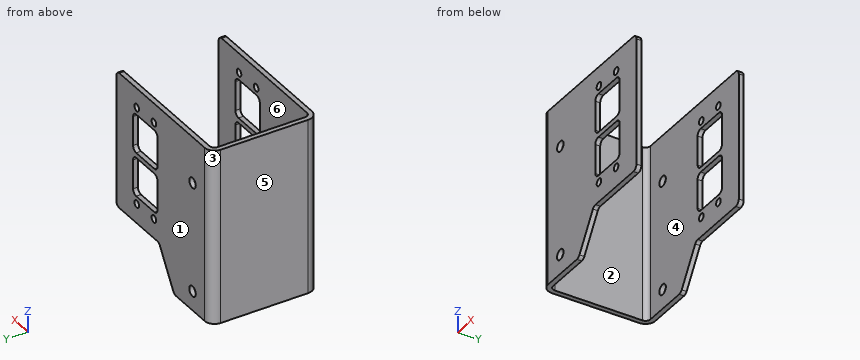
```python
from build123d import *

# Parameters (mm, degrees)
SKETCH1_W                      = 114.3
SKETCH1_H                      = 69.85
BASE_FLANGE1_DEPTH             = 3.175
EDGE_FLANGE1_STRIP_W           = 19.05
EDGE_FLANGE1_STRIP_H           = 3.175
EDGE_FLANGE1_STRIP_CUT_DEPTH   = 114.3
EDGE_FLANGE1_STRIP_2_W         = 19.05
EDGE_FLANGE1_STRIP_2_H         = 3.175
EDGE_FLANGE1_STRIP_CUT_2_DEPTH = 114.3
EDGE_FLANGE1_DEPTH             = 114.3
EDGE_FLANGE1_BEND_DEPTH        = 114.3
SKETCH12_R                     = 2.38125
SKETCH12_R_2                   = 3.3734375
CUT_EXTRUDE1_DEPTH             = 165.36567464
FILLET1_R                      = 3.175


# Sheet-metal steps are written as plain solids
with BuildPart() as part:
    # Sketch1 → Base-Flange1 (new body)
    with BuildSketch(Plane(origin=(0, 0, 0), x_dir=(0, 0, -1), z_dir=(1, 0, 0))):
        with Locations((57.15, 34.925)):
            Rectangle(SKETCH1_W, SKETCH1_H)
    extrude(amount=-BASE_FLANGE1_DEPTH)

    # Edge-Flange1 strip (across the edge) → Edge-Flange1 strip cut (cut)
    with BuildSketch(Plane(origin=(0, 69.85, -114.3), x_dir=(0, -1, 0), z_dir=(0, 0, 1))):
        with Locations((-3.175, -1.5875)):
            Rectangle(EDGE_FLANGE1_STRIP_W, EDGE_FLANGE1_STRIP_H)
    extrude(amount=EDGE_FLANGE1_STRIP_CUT_DEPTH, mode=Mode.SUBTRACT)

    # Edge-Flange1 strip 2 (across the edge) → Edge-Flange1 strip cut 2 (cut)
    with BuildSketch(Plane.YX):
        with Locations((-3.175, -1.5875)):
            Rectangle(EDGE_FLANGE1_STRIP_2_W, EDGE_FLANGE1_STRIP_2_H)
    extrude(amount=EDGE_FLANGE1_STRIP_CUT_2_DEPTH, mode=Mode.SUBTRACT)

    # Edge-Flange1 section (across the edge) → Edge-Flange1 (add)
    with BuildSketch(Plane(origin=(0, 69.85, -114.3), x_dir=(0, -1, 0), z_dir=(0, 0, 1))):
        with BuildLine():
            Line((0, 3.175), (0, 95.25))
            Line((0, 95.25), (3.175, 95.25))
            Line((3.175, 95.25), (3.175, 3.175))
            ThreePointArc((3.175, 3.175), (4.10493597, 0.92993597), (6.35, 0))
            Line((6.35, 0), (6.35, -3.175))
            ThreePointArc((6.35, -3.175), (1.859871939, -1.315128061), (0, 3.175))
        make_face()
    extrude(amount=EDGE_FLANGE1_DEPTH)

    # Edge-Flange1 section 2 (across the edge) → Edge-Flange1 bend (add)
    with BuildSketch(Plane.YX):
        with BuildLine():
            Line((0, 3.175), (0, 95.25))
            Line((0, 95.25), (3.175, 95.25))
            Line((3.175, 95.25), (3.175, 3.175))
            ThreePointArc((3.175, 3.175), (4.10493597, 0.92993597), (6.35, 0))
            Line((6.35, 0), (6.35, -3.175))
            ThreePointArc((6.35, -3.175), (1.859871939, -1.315128061), (0, 3.175))
        make_face()
    extrude(amount=EDGE_FLANGE1_BEND_DEPTH)

    # Sketch12 → Cut-Extrude1 (cut, through all)
    with BuildSketch(Plane(origin=(0, 69.85, 0), x_dir=(1, 0, 0), z_dir=(0, 1, 0))):
        with Locations(Location((56.1594, 76.2, 0), (0, 0, 180))):
            Circle(SKETCH12_R)
        with Locations(Location((74.01814, 76.2, 0), (0, 0, 180))):
            Circle(SKETCH12_R)
        with Locations(Location((56.1594, 12.7, 0), (0, 0, 180))):
            Circle(SKETCH12_R)
        with Locations(Location((74.01814, 12.7, 0), (0, 0, 180))):
            Circle(SKETCH12_R)
        with Locations(Location((15.875, 101.6, 0), (0, 0, 180))):
            Circle(SKETCH12_R_2)
        with Locations(Location((15.875, 30.226, 0), (0, 0, 180))):
            Circle(SKETCH12_R_2)
        Polygon((34.925, 114.3), (50.8, 88.9), (95.25, 88.9), (95.25, 114.3), align=None)
        with BuildLine():
            Line((55.5625, 71.4375), (74.6125, 71.4375))
            ThreePointArc((74.6125, 71.4375), (76.85756403, 70.50756403), (77.7875, 68.2625))
            Line((77.7875, 68.2625), (77.7875, 49.2125))
            ThreePointArc((77.7875, 49.2125), (76.85756403, 46.96743597), (74.6125, 46.0375))
            Line((74.6125, 46.0375), (55.5625, 46.0375))
            ThreePointArc((55.5625, 46.0375), (53.31743597, 46.96743597), (52.3875, 49.2125))
            Line((52.3875, 49.2125), (52.3875, 68.2625))
            ThreePointArc((52.3875, 68.2625), (53.31743597, 70.50756403), (55.5625, 71.4375))
        make_face()
        with BuildLine():
            Line((74.6125, 42.8625), (55.5625, 42.8625))
            ThreePointArc((55.5625, 42.8625), (53.31743597, 41.93256403), (52.3875, 39.6875))
            Line((52.3875, 39.6875), (52.3875, 20.6375))
            ThreePointArc((52.3875, 20.6375), (53.31743597, 18.39243597), (55.5625, 17.4625))
            Line((55.5625, 17.4625), (74.6125, 17.4625))
            ThreePointArc((74.6125, 17.4625), (76.85756403, 18.39243597), (77.7875, 20.6375))
            Line((77.7875, 20.6375), (77.7875, 39.6875))
            ThreePointArc((77.7875, 39.6875), (76.85756403, 41.93256403), (74.6125, 42.8625))
        make_face()
    extrude(amount=-CUT_EXTRUDE1_DEPTH, mode=Mode.SUBTRACT)

    # Fillet1
    fillet1_edges = [part.edges().sort_by_distance(p)[0] for p in [
        (50.8, 68.2625, -88.9),
        (34.925, 68.2625, -114.3),
        (95.25, 68.2625, -88.9),
        (34.925, 1.5875, -114.3),
        (95.25, 1.5875, -88.9),
        (50.8, 1.5875, -88.9),
        (95.25, 68.2625, 0),
        (95.25, 1.5875, 0),
    ]]
    fillet(fillet1_edges, radius=FILLET1_R)


solid = part.part
```
Input: part model. Units: mm. Frame: model coordinates. Face numbers are marked on the shaded views. A direction names the side the tool comes from. Coordinates: 2 decimals unless noted, no trailing zeros. Write each loop counter-clockwise with the first axis right and the second up, starting at its lowest first coordinate (ties: lowest second). Pieces come first, ordered by that corner, then holes.
1) Set-up query: the marked faces 1 and 2. Return all of +Z, -Z, +X, -X, +Y, -Y with unobstructed straight access to the full face (end or side cutting, diameter ignored); none if empty.
2) Pin query (flat end, axial travel): pin 1 Ø2.5 at (y, z) = (67.5, -31.5) entering from -X; pin 2 Ø4 at (x, z) = (56.16, -12.7) entering from -Y; pin 3 Ø1 at (y, z) = (2, -34.5) entering from -X; pin 4 Ø1.5 at (y, z) = (13, -13.5) entering from +X. Return the tip coordinate at first contact, or that it passes through.
3) Section C-C on x = 41. Output: boundary loops of the cut face in (y, z) (3 decimals), and give its area (3 significant figures).
4) Section B-B on z = -12.7. Output: boundary loops of the cut face in (x, y) (3 decimals), and give its area (3 significant figures).
5) Material intervals for line 1 along Y through (x, z) = (36, -97) (3 decimals); line 2 along X through (y, z) = (67, -76); line 3 along X through (y, z) = (68, -12), sorted ascending.
6) Section A-A on x = 61. State how many separate pieces and enclosed holes the cut face has, and give its area (3 significant figures).
7) Mould query, pull axis Y, two halves, no side actions, for the marked faces 3, 4, 5 and 6. Classes: pulls with the +Y half, pulls with the -Y half, needs draft (parallel to the pull), parting line crosses it, or undercut.
Check result:
1. face 1: +Z, -Z, +X, -X, +Y
1. face 2: +Z, -Z, +X
2. pin 1: stops at x = -2.55
2. pin 2: passes through
2. pin 3: stops at x = -1.87
2. pin 4: stops at x = 0
3. outline: (0, -104.58) - (3.175, -104.58) - (3.175, 0) - (0, 0) - close; (66.675, -104.58) - (69.85, -104.58) - (69.85, 0) - (66.675, 0) - close
3. area: 664 mm2
4. outline: (-3.175, 6.35) arc R6.35 ccw to (3.175, 0) - (53.778, 0) - (53.778, 3.175) - (3.175, 3.175) arc R3.175 cw to (0, 6.35) - (0, 63.5) arc R3.175 cw to (3.175, 66.675) - (53.778, 66.675) - (53.778, 69.85) - (3.175, 69.85) arc R6.35 ccw to (-3.175, 63.5) - close; (58.541, 0) - (71.637, 0) - (71.637, 3.175) - (58.541, 3.175) - close; (58.541, 66.675) - (71.637, 66.675) - (71.637, 69.85) - (58.541, 69.85) - close; (76.399, 0) - (95.25, 0) - (95.25, 3.175) - (76.399, 3.175) - close; (76.399, 66.675) - (95.25, 66.675) - (95.25, 69.85) - (76.399, 69.85) - close
4. area: 753 mm2
5. line 1: y = 0 to 3.175, 66.675 to 69.85
5. line 2: x = -2.12 to 53.79, 58.53 to 71.65, 76.39 to 95.25
5. line 3: x = -1.31 to 53.88, 58.44 to 71.74, 76.29 to 95.25
6. separate pieces: 6
6. enclosed holes: 0
6. area: 242 mm2
7. face 3: pulls with the +Y half
7. face 4: undercut
7. face 5: needs draft
7. face 6: undercut
